from build123d import *

# Parameters (mm, degrees)
SKETCH1_W                 = 107.15625
SKETCH1_H                 = 1092.2
BASE_FLANGE1_DEPTH        = 3.175
EDGE_FLANGE1_DEPTH        = 711.2
EDGE_FLANGE1_BEND_DEPTH   = 711.2
F_1_4_CLEARANCE_HOLE1_D   = 6.7564
FILLET3_R                 = 12.7
FILLET4_R                 = 25.4
F_1_START                 = -3.175
F_1_1_5_DOWEL_SLOT1_DEPTH = 3.175
SKETCH25_W                = 25.4
SKETCH25_H                = 4.7625
CUT_EXTRUDE1_DEPTH        = 551.697920975
FILLET5_R                 = 0.79375
FILLET6_R                 = 1.5875
FILLET5_OF_MIRROR1_R      = 0.79375
FILLET6_OF_MIRROR1_R      = 1.5875


# Read off the part's stored shape, not the designer's step: 1 (1.5) Dowel Slot1
# Sheet-metal steps are written as plain solids
with BuildPart() as part:
    # Sketch1 → Base-Flange1 (new body)
    with BuildSketch(Plane.XY):
        Rectangle(SKETCH1_W, SKETCH1_H)
    extrude(amount=-BASE_FLANGE1_DEPTH)

    # Edge-Flange1 section (across the edge) → Edge-Flange1 (add)
    with BuildSketch(Plane(origin=(56.753125, 355.6, -3.175), x_dir=(-1, 0, 0), z_dir=(0, -1, 0))):
        with BuildLine():
            Line((-3.175, 3.175), (-3.175, 34.925))
            Line((-3.175, 34.925), (0, 34.925))
            Line((0, 34.925), (0, 3.175))
            ThreePointArc((0, 3.175), (0.92993597, 0.92993597), (3.175, 0))
            Line((3.175, 0), (3.175, -3.175))
            ThreePointArc((3.175, -3.175), (-1.315128061, -1.315128061), (-3.175, 3.175))
        make_face()
    extrude(amount=EDGE_FLANGE1_DEPTH)

    # Edge-Flange1 section 2 (across the edge) → Edge-Flange1 bend (add)
    with BuildSketch(Plane(origin=(-56.753125, -355.6, -3.175), x_dir=(1, 0, 0), z_dir=(0, 1, 0))):
        with BuildLine():
            Line((-3.175, 3.175), (-3.175, 34.925))
            Line((-3.175, 34.925), (0, 34.925))
            Line((0, 34.925), (0, 3.175))
            ThreePointArc((0, 3.175), (0.92993597, 0.92993597), (3.175, 0))
            Line((3.175, 0), (3.175, -3.175))
            ThreePointArc((3.175, -3.175), (-1.315128061, -1.315128061), (-3.175, 3.175))
        make_face()
    extrude(amount=EDGE_FLANGE1_BEND_DEPTH)

    # 1/4 Clearance Hole1 (through all)
    with Locations(Plane(origin=(59.928125, 0, 0), x_dir=(0, 0, -1), z_dir=(1, 0, 0))):
        with Locations((22.225, 330.2), (22.225, -330.2)):
            Hole(F_1_4_CLEARANCE_HOLE1_D / 2)

    # Fillet3
    fillet3_edges = [part.edges().sort_by_distance(p)[0] for p in [
        (58.340625, 355.6, -38.1),
        (58.340625, -355.6, -38.1),
        (-58.340625, -355.6, -38.1),
        (-58.340625, 355.6, -38.1),
    ]]
    fillet(fillet3_edges, radius=FILLET3_R)

    # Fillet4
    fillet4_edges = [part.edges().sort_by_distance(p)[0] for p in [
        (53.578125, -546.1, -1.5875),
        (-53.578125, -546.1, -1.5875),
        (-53.578125, 546.1, -1.5875),
        (53.578125, 546.1, -1.5875),
    ]]
    fillet(fillet4_edges, radius=FILLET4_R)

    # 1 (1.5) Dowel Slot1 outline → 1 (1.5) Dowel Slot1 (cut)
    with BuildSketch(Plane.XY.offset(F_1_START)):
        with BuildLine():
            ThreePointArc((-19.05, 450.85), (0, 431.8), (19.05, 450.85))
            Line((19.05, 450.85), (19.05, 463.55))
            ThreePointArc((19.05, 463.55), (0, 482.6), (-19.05, 463.55))
            Line((-19.05, 463.55), (-19.05, 450.85))
        make_face()
        with BuildLine():
            ThreePointArc((-19.05, -463.55), (0, -482.6), (19.05, -463.55))
            Line((19.05, -463.55), (19.05, -450.85))
            ThreePointArc((19.05, -450.85), (0, -431.8), (-19.05, -450.85))
            Line((-19.05, -450.85), (-19.05, -463.55))
        make_face()
    extrude(amount=F_1_1_5_DOWEL_SLOT1_DEPTH, mode=Mode.SUBTRACT)

    # Sketch25 → Cut-Extrude1 (cut, through all)
    with BuildSketch(Plane.XY):
        with Locations((-34.528125, 190.5)):
            Rectangle(SKETCH25_W, SKETCH25_H)
        Polygon((0, 193.59332287), (6.35, 183.35625), (3.175, 183.35625), (3.175, 168.19332287), (-3.175, 168.19332287), (-3.175, 183.35625), (-6.35, 183.35625), align=None)
        with Locations((34.528125, 190.5)):
            Rectangle(SKETCH25_W, SKETCH25_H)
    cut_extrude1 = extrude(amount=-CUT_EXTRUDE1_DEPTH, mode=Mode.SUBTRACT)

    # Fillet5
    fillet5_edges = [part.edges().sort_by_distance(p)[0] for p in [
        (-6.35, 183.35625, -1.5875),
        (0, 193.59332287, -1.5875),
        (6.35, 183.35625, -1.5875),
        (3.175, 183.35625, -1.5875),
        (3.175, 168.19332287, -1.5875),
        (-3.175, 168.19332287, -1.5875),
        (-3.175, 183.35625, -1.5875),
    ]]
    fillet(fillet5_edges, radius=FILLET5_R)

    # Fillet6
    fillet6_edges = [part.edges().sort_by_distance(p)[0] for p in [
        (-47.228125, 188.11875, -1.5875),
        (-47.228125, 192.88125, -1.5875),
        (-21.828125, 192.88125, -1.5875),
        (-21.828125, 188.11875, -1.5875),
        (47.228125, 192.88125, -1.5875),
        (47.228125, 188.11875, -1.5875),
        (21.828125, 188.11875, -1.5875),
        (21.828125, 192.88125, -1.5875),
    ]]
    fillet(fillet6_edges, radius=FILLET6_R)

    # Mirror1: Cut-Extrude1 across plane
    add(cut_extrude1.mirror(Plane.ZX), mode=Mode.SUBTRACT)

    # Fillet5 of Mirror1
    fillet5_of_mirror1_edges = [part.edges().sort_by_distance(p)[0] for p in [
        (-6.35, -183.35625, -1.5875),
        (0, -193.59332287, -1.5875),
        (6.35, -183.35625, -1.5875),
        (3.175, -183.35625, -1.5875),
        (3.175, -168.19332287, -1.5875),
        (-3.175, -168.19332287, -1.5875),
        (-3.175, -183.35625, -1.5875),
    ]]
    fillet(fillet5_of_mirror1_edges, radius=FILLET5_OF_MIRROR1_R)

    # Fillet6 of Mirror1
    fillet6_of_mirror1_edges = [part.edges().sort_by_distance(p)[0] for p in [
        (-47.228125, -188.11875, -1.5875),
        (-47.228125, -192.88125, -1.5875),
        (-21.828125, -192.88125, -1.5875),
        (-21.828125, -188.11875, -1.5875),
        (47.228125, -192.88125, -1.5875),
        (47.228125, -188.11875, -1.5875),
        (21.828125, -188.11875, -1.5875),
        (21.828125, -192.88125, -1.5875),
    ]]
    fillet(fillet6_of_mirror1_edges, radius=FILLET6_OF_MIRROR1_R)


solid = part.part
Source: CAD feature listing. Evaluate the final solid. Frame: model axes, mm. A direction names the side the tool comes from. Coordinates: 2 decimals unless noted, no trailing zeros. Loops run counter-clockwise (first coordinate to the right, second up) from the corner with the lowest first, then second, coordinate; pieces in that order, holes last. Notation, with made-up numbers: (89, 75) - (104, 75) arc R31 cw to (104, 114) - close; hole circle Ø4 at (-21.75, 61.25). An arc over 180 degrees is marked (long way). Return JSON: item names as keys, results as strings.
Q1. Access query for faces 4 (the flat face through (-1, 8, -3.175)), 5 (the cylindrical face through (-46.3, -538.5, -1.6)), 6 (the cylindrical face through (0.419, 482.595, -1.61)). Directions: +Z, -Z, +X, -X, +Y, -Y. A direction counts if a zero-diameter tool reaches every point of the face in a straight line with its end or side. Return the directions, or none.
Results:
{"face 4": "-Z, +Y, -Y", "face 5": "+Z, -Z, -X, -Y", "face 6": "+Z, -Z"}
Q2. Material intervals for line 1 along X through (y, z) = (-13, -28.5); line 2 along X through (y, z) = (-333, -6); line 3 along Z through (x, y) = (-30, -347.5) (3 decimals), sorted ascending.
Results:
{"line 1": "-59.93 to -56.75, 56.75 to 59.93", "line 2": "-59.92 to -56.73, 56.73 to 59.92", "line 3": "-3.175 to 0"}
Q3. Mould query, pull axis Y, two halves, no side actions, for faces 1 (the flat face through (-56.753, -5, -22)), 2 (the cylindrical face through (-0.419, 431.805, -1.61)), 3 (the cylindrical face through (46.3, 538.5, -1.6)). Classes: released by +Y, released by -Y, zero draft, split by the parting line, or undercut.
Results:
{"face 1": "zero draft", "face 2": "undercut", "face 3": "released by +Y"}
Q4. Contact query for flat-ended pins moving along their axis: P1, Ø5, axis at x = 55, z = -10, coming from the +Y side; P2, Ø3.5, axis at x = 35, z = -2, coming from the +Y side; P3, Ø5, axis at x = -25.5, y = 55, coming from the -Z side (3 decimals). Output: stop coordinate, or through.
Results:
{"P1": "y = 355.6", "P2": "y = 545.59", "P3": "z = -3.175"}
Q5. Section A-A, the plane y = -242.5. Return loops of the section in (x, z) (3 decimals), plus the area to 3 significant figures.
Results:
{"outline": "(-59.928, -38.1) - (-56.753, -38.1) - (-56.753, -6.35) arc R3.175 cw to (-53.578, -3.175) - (53.578, -3.175) arc R3.175 cw to (56.753, -6.35) - (56.753, -38.1) - (59.928, -38.1) - (59.928, -6.35) arc R6.35 ccw to (53.578, 0) - (-53.578, 0) arc R6.35 ccw to (-59.928, -6.35) - close", "area": "589 mm2"}
